The drawing under review shows one solid part. Ordinate dimensions are in mm from its lowest x, y, z. A direction names the side the tool comes from. Round coordinates to 2 decimals unless told otherwise and drop trailing zeros. Order: outer loops, then holes, each group sorted by start corner. A loop starts at its lowest first (then second) coordinate and runs counter-clockwise, first axis right, second up.
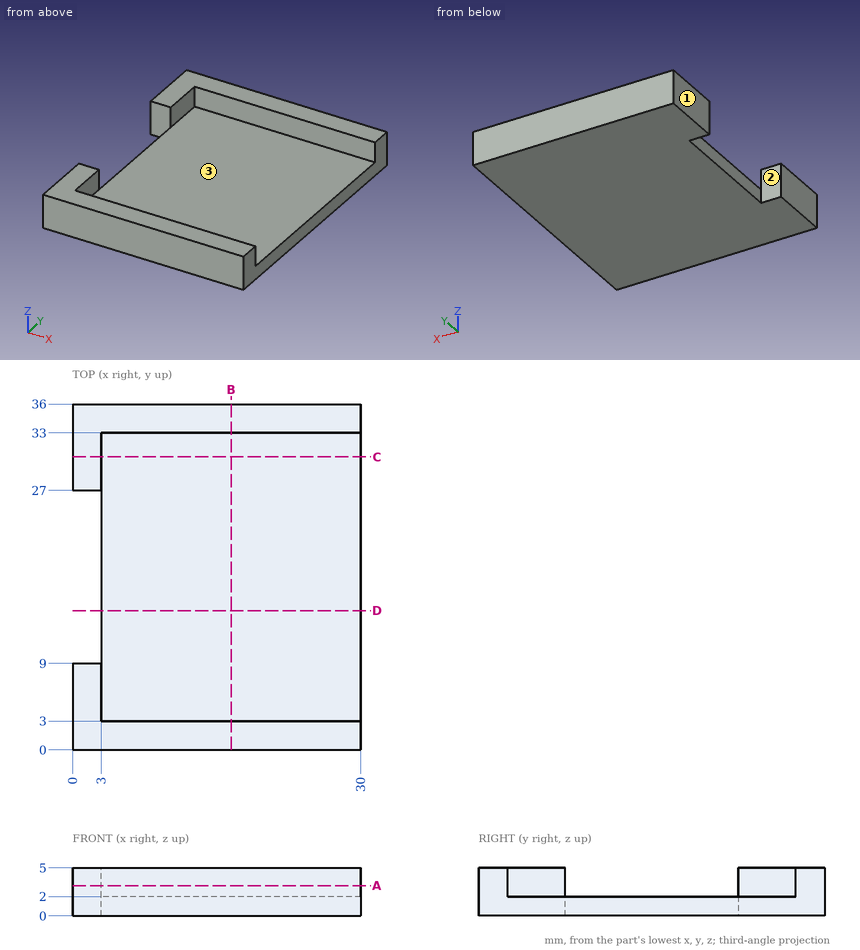
(1) We need section B-B (x = 16.5). Give the boundary of the cut face in (y, z).
(2) Clearance check with flat-ended pins moving along their axes: P1, Ø4, axis at x = 7.5, y = 14.5, coming from the +Z side; P2, Ø1.6, axis at y = 14, z = 1.5, coming from the -X side. State where each tip first meets the part, or that it passes through.
(3) We need section D-D (y = 14.5). Give the boundary of the cut face in (x, z).
(4) We need section C-C (y = 30.5). Give the boundary of the cut face in (x, z), and give its area (3 significant figures).
(5) We need section A-A (z = 3.15). Give the boundary of the cut face in (x, y).
(6) To check wall thickness, follow L1, parallel to Y at x = 7.25, z = 3.25; L2, parallel to Z at x = 28.5, y = 19; L3, parallel to Y at x = 2.5, z = 0.85. State the ranges of each line that lie inside material, in increasing order.
(7) Tool access review of the marked faces 1, 2 and 3: name each direction out of +Z, -Z, +X, -X, +Y, -Y from which nothing blocks a thin tool from reaching the whole face with its end or side.
Verdict:
1. outline: (0, 0) - (36, 0) - (36, 5) - (33, 5) - (33, 2) - (3, 2) - (3, 5) - (0, 5) - close
2. P1: stops at z = 2
2. P2: stops at x = 3
3. outline: (3, 0) - (30, 0) - (30, 2) - (3, 2) - close
4. outline: (0, 0) - (30, 0) - (30, 2) - (3, 2) - (3, 5) - (0, 5) - close
4. area: 69.0 mm2
5. outline: (0, 0) - (30, 0) - (30, 3) - (3, 3) - (3, 9) - (0, 9) - close; (0, 27) - (3, 27) - (3, 33) - (30, 33) - (30, 36) - (0, 36) - close
6. L1: y = 0 to 3, 33 to 36
6. L2: z = 0 to 2
6. L3: y = 0 to 9, 27 to 36
7. face 1: +Z, -Z, -X, +Y, -Y
7. face 2: +Z, -Z, -X
7. face 3: +Z, +X
